Drawing for the job (mm, zero at the part's lowest x, y, z). Round coordinates to 2 decimals unless told otherwise and drop trailing zeros. Write each loop counter-clockwise with the first axis right and the second up, starting at its lowest first coordinate (ties: lowest second). Pieces come first, ordered by that corner, then holes. Notation, with made-up numbers: (39, 21) - (87, 21) arc R25 ccw to (87, 43) - close; hole circle Ø7 at (-14.75, 12). An arc over 180 degrees is marked (long way). Answer in a Markdown table with one row per item.
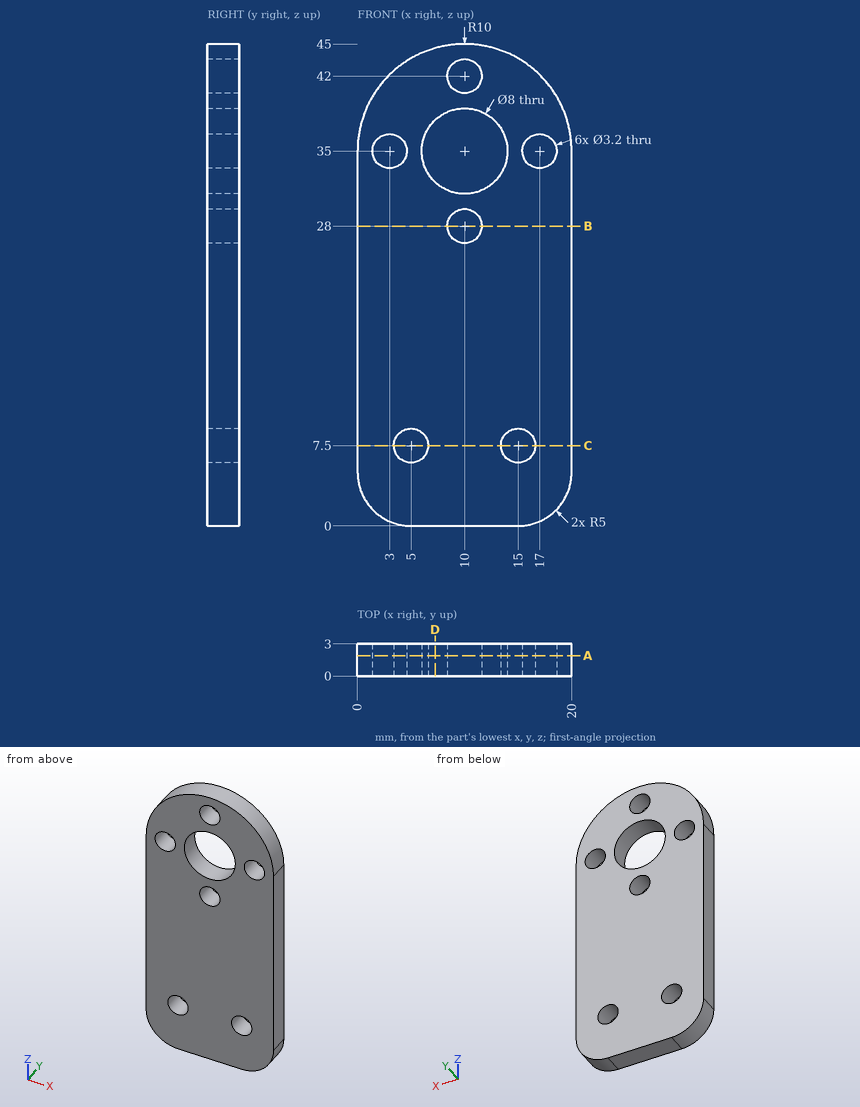
Q1. Saw through at A-A on y = 1.9. List the corners of the cut face in (x, z), then the cut area to 3 significant figures.
Computed:
| item | result |
|---|---|
| outline | (0, 5) arc R5 ccw to (5, 0) - (15, 0) arc R5 ccw to (20, 5) - (20, 35) arc R10 ccw to (0, 35) - close; hole circle Ø3.2 at (3, 35); hole circle Ø3.2 at (5, 7.5); hole circle Ø8 at (10, 35); hole circle Ø3.2 at (10, 28); hole circle Ø3.2 at (10, 42); hole circle Ø3.2 at (15, 7.5); hole circle Ø3.2 at (17, 35) |
| area | 748 mm2 |
Q2. Saw through at B-B on z = 28. List the corners of the cut face in (x, y).
Computed:
| item | result |
|---|---|
| outline | (0, 0) - (8.4, 0) - (8.4, 3) - (0, 3) - close; (11.6, 0) - (20, 0) - (20, 3) - (11.6, 3) - close |
Q3. Saw through at D-D on x = 7.25. List the corners of the cut face in (y, z).
Computed:
| item | result |
|---|---|
| outline | (0, 0) - (3, 0) - (3, 32.1) - (0, 32.1) - close; (0, 37.9) - (3, 37.9) - (3, 44.61) - (0, 44.61) - close |
Q4. Drill centre lines: line 1 (X direction, y = 1.5, z = 35); line 2 (X direction, y = 1.85, z = 7.5); line 3 (X direction, y = 2.2, z = 28). Where is each one in solid material? Low to high.
Computed:
| item | result |
|---|---|
| line 1 | x = 0 to 1.4, 4.6 to 6, 14 to 15.4, 18.6 to 20 |
| line 2 | x = 0 to 3.4, 6.6 to 13.4, 16.6 to 20 |
| line 3 | x = 0 to 8.4, 11.6 to 20 |
Q5. Saw through at C-C on z = 7.5. List the corners of the cut face in (x, y), then the cut area to 3 significant figures.
Computed:
| item | result |
|---|---|
| outline | (0, 0) - (3.4, 0) - (3.4, 3) - (0, 3) - close; (6.6, 0) - (13.4, 0) - (13.4, 3) - (6.6, 3) - close; (16.6, 0) - (20, 0) - (20, 3) - (16.6, 3) - close |
| area | 40.8 mm2 |
Q6. Flat gauge pins, fed straight in: pin 1 (2.5 mm diameter, centred on x = 17, z = 35, fed in from -Y); pin 2 (1.5 mm diameter, centred on x = 17.5, y = 0.5, fed in from -Z). Where does each tip first touch, or does it go through?
Computed:
| item | result |
|---|---|
| pin 1 | passes through |
| pin 2 | stops at z = 0.32 |
